from build123d import *

# Parameters (mm, degrees)
SKETCH1_W           = 4
SKETCH1_H           = 16
BOSS_EXTRUDE1_DEPTH = 11
SKETCH2_W           = 20
SKETCH2_H           = 20
BOSS_EXTRUDE2_DEPTH = 7
SKETCH3_W           = 20
SKETCH3_H           = 16
SKETCH3_W_2         = 16
SKETCH3_H_2         = 20
BOSS_EXTRUDE3_DEPTH = 3
FILLET1_R           = 2
SKETCH4_R           = 2.5
CUT_EXTRUDE1_DEPTH  = 10
SKETCH5_R           = 4.25
CUT_EXTRUDE2_DEPTH  = 5.2
SKETCH6_R           = 2
CUT_EXTRUDE3_DEPTH  = 5.2


with BuildPart() as part:
    # Sketch1 → Boss-Extrude1 (new body)
    with BuildSketch(Plane(origin=(0, 0, 0), x_dir=(1, 0, 0), z_dir=(0, 1, 0))):
        Polygon((-10, 10), (-6, 10), (-6, 14), (-6, 30), (-10, 30), align=None)
        Polygon((-6, 10), (10, 10), (14, 10), (14, 14), (-6, 14), align=None)
        with Locations((12, 2)):
            Rectangle(SKETCH1_W, SKETCH1_H)
        Polygon((10, -6), (10, -10), (30, -10), (30, -6), (14, -6), align=None)
    extrude(amount=BOSS_EXTRUDE1_DEPTH)

    # Sketch2 → Boss-Extrude2 (add)
    with BuildSketch(Plane(origin=(0, 0, 0), x_dir=(1, 0, 0), z_dir=(0, 1, 0))):
        Rectangle(SKETCH2_W, SKETCH2_H)
    extrude(amount=BOSS_EXTRUDE2_DEPTH)

    # Sketch3 → Boss-Extrude3 (add)
    with BuildSketch(Plane(origin=(0, 11, 0), x_dir=(1, 0, 0), z_dir=(0, 1, 0))):
        with Locations((4, 22)):
            Rectangle(SKETCH3_W, SKETCH3_H)
        with BuildLine():
            Line((30, 14), (14, 14))
            Line((14, 14), (14, 30))
            ThreePointArc((14, 30), (25.313708499, 25.313708499), (30, 14))
        make_face()
        with Locations((22, 4)):
            Rectangle(SKETCH3_W_2, SKETCH3_H_2)
    extrude(amount=-BOSS_EXTRUDE3_DEPTH)

    # Fillet1
    fillet1_edges = [part.edges().sort_by_distance(p)[0] for p in [
        (-6, 4, -30),
        (-6, 4, -14),
        (14, 4, -14),
        (14, 4, 6),
        (30, 4, 6),
        (25.313708499, 8, -25.313708499),
        (30, 8, -4),
        (4, 8, -14),
        (-6, 8, -22),
        (4, 8, -30),
        (22, 8, 6),
        (14, 8, -4),
    ]]
    fillet(fillet1_edges, radius=FILLET1_R)

    # Sketch4 → Cut-Extrude1 (cut)
    with BuildSketch(Plane.XZ):
        with Locations(Location((0, 0, 0), (0, 0, 270))):
            Circle(SKETCH4_R)
    extrude(amount=-CUT_EXTRUDE1_DEPTH, mode=Mode.SUBTRACT)

    # Sketch5 → Cut-Extrude2 (cut)
    with BuildSketch(Plane.XZ):
        with Locations(Location((0, 0, 0), (0, 0, 270))):
            Circle(SKETCH5_R)
    extrude(amount=-CUT_EXTRUDE2_DEPTH, mode=Mode.SUBTRACT)

    # Sketch6 → Cut-Extrude3 (cut)
    with BuildSketch(Plane(origin=(0, 11, 0), x_dir=(1, 0, 0), z_dir=(0, 1, 0))):
        with Locations(Location((22.489995997, 0, 0), (0, 0, 270))):
            Circle(SKETCH6_R)
        with Locations(Location((0, 22.489995997, 0), (0, 0, 270))):
            Circle(SKETCH6_R)
        with Locations(Location((18.838834765, 18.838834765, 0), (0, 0, 270))):
            Circle(SKETCH6_R)
    extrude(amount=-CUT_EXTRUDE3_DEPTH, mode=Mode.SUBTRACT)


solid = part.part
Input: part model. Units: mm. Frame: model coordinates. A direction names the side the tool comes from. Give positions to 0.01 mm unless a question says otherwise; leave off trailing zeros. Write each loop counter-clockwise with the first axis right and the second up, starting at its lowest first coordinate (ties: lowest second). Pieces come first, ordered by that corner, then holes.
Q1. Material intervals for probe 1 along X at (y, z) = (4.05, 0); probe 2 along X at (y, z) = (2.5, -4.5); probe 3 along Y at (x, z) = (9, -26), sorted ascending.
Q2. First-contact query: P1, Ø3, axis at x = -4.5, y = 9, coming from the +Z side; P2, Ø5, axis at x = 0, z = -22.49, coming from the -Y side; P3, Ø3.5, axis at x = 18.84, z = -18.84, coming from the +Y side; P4, Ø6.5, axis at y = 3.5, z = -23, coming from the +X side. Flat tips, straight axial feed; report the tip coordinate or a pass-through.
Q3. Section B-B, the plane x = 0. Output: boundary loops of the cut face in (y, z).
Q4. Set-up query: faces 1 (the face through (4.11, 7.43, -14.6)), 2 (the face through (-2, 7, 2)), 3 (the face through (30, 10.4, 2.5)). Return all of +Z, -Z, +X, -X, +Y, -Y with unobstructed straight access to the full face (end or side cutting, diameter ignored); none if empty.
Q5. Section C-C, the plane y = 2. Output: boundary loops of the cut face in (x, z).
Q6. Pull-direction query (Z, two-part tool) for faces 4 (the face through (10, 11, -15)), 5 (the face through (0.088, 9.521, -24.488)), 6 (the face through (0, 9, -10)), 7 (the face through (13.43, 3.04, -13.4)); classes: pulls with the +Z half, pulls with the -Z half, needs draft (parallel to the pull), parting line crosses it, or undercut.
Q7. Section A-A, the plane z = 0. Output: boundary loops of the cut face in (x, y), plus the area to 3 significant figures.
Filled in:
1. probe 1: x = -10 to -4.25, 4.25 to 14
1. probe 2: x = -10 to 14
1. probe 3: y = 8 to 11
2. P1: stops at z = -10
2. P2: stops at y = 8
2. P3: passes through
2. P4: stops at x = -5.85
3. outline: (0, -14) - (6, -14) arc R2 cw to (8, -16) - (8, -20.49) - (11, -20.49) - (11, -10) - (7, -10) - (7, -2.5) - (5.2, -2.5) - (5.2, -4.25) - (0, -4.25) - close; (0, 4.25) - (5.2, 4.25) - (5.2, 2.5) - (7, 2.5) - (7, 10) - (0, 10) - close; (8, -28) arc R2 ccw to (10, -30) - (11, -30) - (11, -24.49) - (8, -24.49) - close
4. face 1: -Z, +X, -Y
4. face 2: +Z, -X, +Y
4. face 3: +Z, -Z, +X, +Y, -Y
5. outline: (-10, -30) - (-8, -30) arc R2 ccw to (-6, -28) - (-6, -16) arc R2 cw to (-4, -14) - (12, -14) arc R2 ccw to (14, -12) - (14, 4) arc R2 cw to (16, 6) - (28, 6) arc R2 ccw to (30, 8) - (30, 10) - (-10, 10) - close; hole circle Ø8.5 at (0, 0)
6. face 4: needs draft
6. face 5: undercut
6. face 6: pulls with the +Z half
6. face 7: pulls with the -Z half
7. outline: (-10, 0) - (-4.25, 0) - (-4.25, 5.2) - (-2.5, 5.2) - (-2.5, 7) - (-10, 7) - close; (2.5, 5.2) - (4.25, 5.2) - (4.25, 0) - (14, 0) - (14, 6) arc R2 cw to (16, 8) - (20.49, 8) - (20.49, 11) - (10, 11) - (10, 7) - (2.5, 7) - close; (24.49, 8) - (28, 8) arc R2 ccw to (30, 10) - (30, 11) - (24.49, 11) - close
7. area: 167 mm2
